```python
from build123d import *

# Parameters (mm, degrees)
BOSS_EXTRUDE1_DEPTH             = 101.6
FILLET1_R                       = 5.715
F_1_4_0_25_DIAMETER_HOLE1_D     = 6.35
F_1_4_0_25_DIAMETER_HOLE1_DEPTH = 3.4544
LPATTERN1_COUNT                 = 2
LPATTERN1_PITCH                 = 12.7
LPATTERN1_COUNT_DIR2            = 8
LPATTERN1_PITCH_DIR2            = 12.7


with BuildPart() as part:
    # Sketch1 → Boss-Extrude1 (new body, symmetric)
    with BuildSketch(Plane(origin=(0, 0, 0), x_dir=(1, 0, 0), z_dir=(0, 1, 0))):
        Polygon((0, 0), (-26.940768363, -26.940768363), (-24.498138698, -29.383398028), (0, -4.88525933), (24.498138698, -29.383398028), (26.940768363, -26.940768363), align=None)
    extrude(amount=BOSS_EXTRUDE1_DEPTH, both=True)

    # Fillet1
    fillet1_edges = [part.edges().sort_by_distance(p)[0] for p in [
        (0, 0, 4.88525933),
    ]]
    fillet(fillet1_edges, radius=FILLET1_R)

    # 1/4 (0.25) Diameter Hole1
    with Locations(Plane(origin=(2.442629665, 0, 2.442629665), x_dir=(0.707106781, 0, -0.707106781), z_dir=(0.707106781, 0, 0.707106781))):
        with Locations((-28.575, 0)):
            f_1_4_0_25_diameter_hole1 = Hole(F_1_4_0_25_DIAMETER_HOLE1_D / 2, depth=F_1_4_0_25_DIAMETER_HOLE1_DEPTH)

    # LPattern1: 1_4 _0.25_ Diameter Hole1 2 × 8
    with Locations(*[Vector(0.707106781, 0, -0.707106781) * (i * LPATTERN1_PITCH) + Vector(0, -1, 0) * (j * LPATTERN1_PITCH_DIR2) for i in range(LPATTERN1_COUNT) for j in range(LPATTERN1_COUNT_DIR2) if (i, j) != (0, 0)]):
        add(f_1_4_0_25_diameter_hole1, mode=Mode.SUBTRACT)


solid = part.part
```
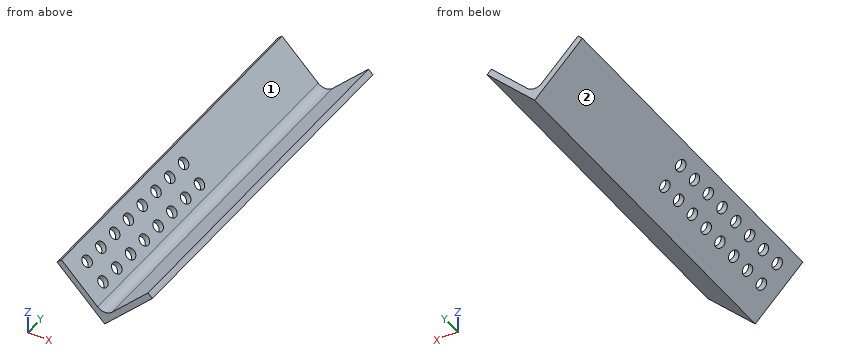
Can you work these out from the model? Positions are in its coordinate system, mm. Face numbers are marked on the shaded views. A direction names the side the tool comes from. Round coordinates to 2 decimals unless told otherwise and drop trailing zeros. Order: outer loops, then holes, each group sorted by start corner. A loop starts at its lowest first (then second) coordinate and runs counter-clockwise, first axis right, second up.
(1) If we section it at A-A (y = -58.5): Please give me the cut outline in (x, z) (3 decimals), plus the area to 3 significant figures.
Results are:
outline: (-26.941, 26.941) - (0, 0) - (26.941, 26.941) - (24.498, 29.383) - (4.041, 8.926) arc R5.715 cw to (-4.041, 8.926) - (-24.498, 29.383) - close
area: 258 mm2
(2) If I drill on L1, parallel to X at y = 5, z = 15.5; L2, parallel to X at y = -65, z = 28.25; L3, parallel to Z at x = -4, y = -19, over which ranges is the centre line in solid material (lowest first)?
Results are:
L1: x = -15.5 to -10.61, 10.61 to 15.5
L2: x = -25.63 to -23.36, 23.36 to 25.63
L3: z = 4 to 8.89
(3) I'm going to push flat-ended pins straight in: pin 1 (10 mm diameter, centred on y = -67.5, z = 18.5, fed in from -X); pin 2 (10 mm diameter, centred on y = 67, z = 17, fed in from -X); pin 3 (1 mm diameter, centred on y = 55.5, z = 26, fed in from +X). Where does each tip first touch, or does it pass through?
Results are:
pin 1: stops at x = -23.5
pin 2: stops at x = -22
pin 3: stops at x = 26.5
(4) If we section it at B-B (z = 2.75): Please give me the cut outline in (x, y), plus the area to 3 significant figures.
Results are:
outline: (-2.75, -101.6) - (2.75, -101.6) - (2.75, 101.6) - (-2.75, 101.6) - close
area: 1,120 mm2
(5) If we section it at C-C (x = 18): Please give me the cut outline in (y, z), plus the area to 3 significant figures.
Results are:
outline: (-101.6, 18) - (101.6, 18) - (101.6, 22.89) - (-101.6, 22.89) - close
area: 993 mm2
(6) On a 3-axis mill with a long thin cutter (end or side, diameter ignored), from which of +Z, -Z, +X, -X, +Y, -Y can I reach the whole of each face in a straight line? I mean the marked faces 1 and 2. Say none if no direction works.
Results are:
face 1: +Z, +Y, -Y
face 2: -Z, -X, +Y, -Y
